Autodesk Inventor part; units mm, degrees
ref_plane "YZ Plane" through (0, 0, 0) normal (1, 0, 0) x (0, 1, 0)
ref_plane "XZ Plane" through (0, 0, 0) normal (0, 1, 0) x (-1, 0, 0)
ref_plane "XY Plane" through (0, 0, 0) normal (0, 0, 1) x (1, 0, 0)
sketch "Sketch1" plane through (0, 0, 0) normal (0, 1, 0) x (-1, 0, 0)
  line L0 (0, 0) -> (-177.8, 0)
  line L1 (-177.8, 0) -> (-177.8, -76.2)
  line L2 (-177.8, -76.2) -> (0, -76.2)
  line L3 (0, -76.2) -> (0, 0)
  dimension "d0" = 177.8
  dimension "d1" = 76.2
extrude "Extrusion1" add sketch "Sketch1" along normal blind 165.1
sketch "Sketch2" plane through (0, 165.1, 0) normal (0, 1, 0) x (1, 0, 0)
  line L0 (177.8, 25.4) -> (130.175, 25.4)
  line L1 (130.175, 25.4) -> (130.175, 0)
  line L2 (0, 25.4) -> (47.625, 25.4)
  line L3 (47.625, 25.4) -> (47.625, 0)
  line L4 (0, 0) -> (177.8, 0)
  line L5 (0, 76.2) -> (0, 0)
  line L6 (177.8, 0) -> (177.8, 76.2)
  line L7 (0, 25.4) -> (0, 0)
  line L8 (0, 0) -> (47.625, 0)
  line L9 (130.175, 0) -> (177.8, 0)
  line L10 (177.8, 25.4) -> (177.8, 0)
  dimension "d4" = 47.625
  dimension "d5" = 47.625
  dimension "d6" = 25.4
  dimension "d7" = 25.4
extrude "Extrusion2" cut sketch "Sketch2" against normal blind 12.7
properties part number "Battery"
Build history of the part. All positions in model axes, mm. A direction names the side the tool comes from. Give positions to 0.01 mm unless a question says otherwise; leave off trailing zeros. Loops run counter-clockwise (first coordinate to the right, second up) from the corner with the lowest first, then second, coordinate; pieces in that order, holes last. Notation, with made-up numbers: (41, 70) - (46, 70) arc R18 ccw to (46, 102) - close; hole circle Ø6 at (49.25, 80.25). An arc over 180 degrees is marked (long way). Write item = value, one per line. Start each with the question number.
1) Band-saw the part on B-B on x = 153. Give the cut face in (y, z), plus the area to 3 significant figures.
2) Band-saw the part on A-A on z = -11.5. Give the cut face in (x, y) (3 decimals).
3) Drop flat-ended pins along their axis: pin 1 Ø8 at (x, z) = (35, -20.5) entering from +Y; pin 2 Ø4 at (y, z) = (160.5, -12.5) entering from +X (3 decimals). Give the stop position or say it passes through.
4) Tool access for faces 1 (the flat face through (47.625, 159, -13)), 2 (the flat face through (88, 81, 0)), 3 (the flat face through (154, 159, -25.4)): list every direction of +Z, -Z, +X, -X, +Y, -Y with a clear straight run to the whole face (end or side of a thin tool).
Final values:
q1.outline = (0, -76.2) - (165.1, -76.2) - (165.1, -25.4) - (152.4, -25.4) - (152.4, 0) - (0, 0) - close
q1.area = 12,300 mm²
q2.outline = (0, 0) - (177.8, 0) - (177.8, 152.4) - (130.175, 152.4) - (130.175, 165.1) - (47.625, 165.1) - (47.625, 152.4) - (0, 152.4) - close
q3.pin_1 = 152.4
q3.pin_2 = 130.175
q4.face_1 = +Z, -X, +Y
q4.face_2 = +Z, +X, -X, +Y, -Y
q4.face_3 = +Z, +X, +Y
